```python
from build123d import *
from build123d.topology import SkipClean

# Parameters (mm, degrees)
SKETCH_1_W               = 14
SKETCH_1_H               = 45
EXTRUDE_1_DEPTH          = 3
SKETCH_4_W               = 8
SKETCH_4_H               = 3.5
EXTRUDE_2_DEPTH          = 10
SKETCH_10_W              = 3.5
SKETCH_10_H              = 6
EXTRUDE_3_DEPTH          = 14
CUT_EXTRUDE_1_DEPTH      = 52.078371156
CUT_EXTRUDE_1_DEPTH_BACK = 52.078371156
SKETCH_2_R               = 1.5
SKETCH_3_R               = 3.5
SKETCH_3_R_2             = 1.5
EXTRUDE_1_2_DEPTH        = 5
SKETCH_12_W              = 14
SKETCH_12_H              = 2
EXTRUDE_4_DEPTH          = 5
RIB_9_REACH              = 53.078
SKETCH_13_WALL_W         = 123.475258838
SKETCH_13_WALL_H         = 2.8
RIB_8_REACH              = 53.078
SKETCH_11_WALL_W         = 124.678564032
SKETCH_11_WALL_H         = 3
CHAMFER_3_SIZE           = 0.5
CHAMFER_4_SIZE           = 1
EXTRUDE_5_REACH          = 46.612
EXTRUDE_5_END_RADIUS     = 3.5
SKETCH_15_W              = 5.2
SKETCH_15_H              = 5
CHAMFER_5_SIZE           = 0.606199956
CHAMFER_5_SIZE_2         = 1.3
CUT_EXTRUDE_2_DEPTH      = 4
EXTRUDE_START            = 3
EXTRUDE_6_DEPTH          = 4.393800044
CUT_EXTRUDE_3_DEPTH      = 1
CHAMFER_START            = 2.8
CHAMFER_6_DEPTH          = 2.5
CHAMFER_START_2          = 5.3
CHAMFER_6_2_DEPTH        = 2.7
CHAMFER_START_3          = 3
CHAMFER_6_3_DEPTH        = 3.7
DELETE_START             = 2
DELETE_FACE_1_DEPTH      = 6


with BuildPart() as part:
    # 草图1 → Extrude 1 (new body)
    with BuildSketch(Plane(origin=(0, 0, 0), x_dir=(1, 0, 0), z_dir=(0, 1, 0))):
        with Locations((7, -22.5)):
            Rectangle(SKETCH_1_W, SKETCH_1_H)
    extrude(amount=EXTRUDE_1_DEPTH)

    # 草图4 → 凸台-拉伸2 (add)
    with BuildSketch(Plane.XZ):
        with Locations((18, 1.75)):
            Rectangle(SKETCH_4_W, SKETCH_4_H)
    extrude_2 = extrude(amount=-EXTRUDE_2_DEPTH)

    # 草图9 → 打孔尺寸(%根据)内六角花形半沉头螺钉的类型1 (revolve, cut)
    with BuildSketch(Plane(origin=(18, 5, 3.5), x_dir=(0, -1, 0), z_dir=(1, 0, 0))):
        Polygon((0, 0), (0, 5.96137699), (1.6, 5), (1.6, 1.6), (3.2, 0), align=None)
    hole_wizard_1 = revolve(axis=Axis((18, 5, 9.85), (0, 0, -1)), mode=Mode.SUBTRACT)

    # 镜向1: 凸台-拉伸2, 打孔尺寸(%根据)内六角花形半沉头螺钉的类型1 across plane
    add(extrude_2.mirror(Plane(origin=(7, 0, 0), x_dir=(0, 0, 1), z_dir=(1, 0, 0))))
    add(hole_wizard_1.mirror(Plane(origin=(7, 0, 0), x_dir=(0, 0, 1), z_dir=(1, 0, 0))), mode=Mode.SUBTRACT)

    # 草图10 → 凸台-拉伸3 (add)
    with BuildSketch(Plane.ZY.offset(-14)):
        with Locations((1.75, 6)):
            Rectangle(SKETCH_10_W, SKETCH_10_H)
    extrude(amount=EXTRUDE_3_DEPTH)

    # 草图2 → 切除-拉伸1 (cut, two sides: drawn at the far end of the back side and taken through both)
    with BuildSketch(Plane.XZ.offset(-CUT_EXTRUDE_1_DEPTH_BACK)):
        with Locations(Location((4.5, 41, 0), (0, 0, 270))):
            Circle(SKETCH_2_R)
        with Locations(Location((4.5, 4, 0), (0, 0, 270))):
            Circle(SKETCH_2_R)
    extrude(amount=CUT_EXTRUDE_1_DEPTH + CUT_EXTRUDE_1_DEPTH_BACK, mode=Mode.SUBTRACT)

    # 草图3 → Extrude 1 2 (add)
    # profile 1 of 2: a face of its own
    with SkipClean():  # the faces are left unmerged after this step: merging them gives an invalid solid
        with BuildSketch(Plane(origin=(0, 3, 0), x_dir=(1, 0, 0), z_dir=(0, 1, 0))):
            with Locations((4.5, -41)):
                Circle(SKETCH_3_R)
            with Locations((4.5, -41)):
                Circle(SKETCH_3_R_2, mode=Mode.SUBTRACT)
        # profile 2 of 2: a face of its own
        with BuildSketch(Plane(origin=(0, 3, 0), x_dir=(1, 0, 0), z_dir=(0, 1, 0))):
            with Locations((4.5, -4)):
                Circle(SKETCH_3_R)
            with Locations((4.5, -4)):
                Circle(SKETCH_3_R_2, mode=Mode.SUBTRACT)
        extrude(amount=EXTRUDE_1_2_DEPTH)

    # 草图12 → 凸台-拉伸4 (add)
    with SkipClean():  # the faces are left unmerged after this step: merging them gives an invalid solid
        with BuildSketch(Plane(origin=(0, 3, 0), x_dir=(1, 0, 0), z_dir=(0, 1, 0))):
            with Locations((7, -44)):
                Rectangle(SKETCH_12_W, SKETCH_12_H)
        extrude(amount=EXTRUDE_4_DEPTH)

    # 草图13 wall → 筋9 (add, up to next)
    with BuildSketch(Plane(origin=(14, 5.5, 33.669872981), x_dir=(0, -0.258819045101, -0.96592582629), z_dir=(0, 0.96592582629, -0.258819045101)), mode=Mode.PRIVATE) as rib_9_sk1:
        with Locations((0, 1.4)):
            Rectangle(SKETCH_13_WALL_W, SKETCH_13_WALL_H)
    rib_9_tool1 = extrude(rib_9_sk1.sketch, amount=-RIB_9_REACH, mode=Mode.PRIVATE) - part.part
    rib_9 = rib_9_tool1.solids().sort_by_distance((14, 5.5, 33.669872981))[0]
    add(rib_9)

    # 草图11 wall → 筋8 (add, up to next)
    with BuildSketch(Plane(origin=(14, 6, 13.312557855), x_dir=(0, -0.292371704721, 0.956304755963), z_dir=(0, -0.956304755963, -0.292371704721)), mode=Mode.PRIVATE) as rib_8_sk1:
        with Locations((0, 1.5)):
            Rectangle(SKETCH_11_WALL_W, SKETCH_11_WALL_H)
    rib_8_tool1 = extrude(rib_8_sk1.sketch, amount=RIB_8_REACH, mode=Mode.PRIVATE) - part.part
    rib_8 = rib_8_tool1.solids().sort_by_distance((14, 6, 13.312557855))[0]
    add(rib_8)

    # 镜向2: 筋9, 筋8 across plane
    with SkipClean():  # the faces are left unmerged after this step: merging them gives an invalid solid
        add(rib_9.mirror(Plane(origin=(7, 0, 0), x_dir=(0, 0, 1), z_dir=(1, 0, 0))))
        add(rib_8.mirror(Plane(origin=(7, 0, 0), x_dir=(0, 0, 1), z_dir=(1, 0, 0))))

    # 倒角3
    # the kernel refuses this chamfer: 0.5 mm, written as the material it adds along each edge
    with BuildSketch(Plane(origin=(14, 3, 3.5), x_dir=(1, 0, 0), z_dir=(0, 1, 0))) as chamfer_3_piece_1_section:
        Polygon((CHAMFER_3_SIZE, 0), (0, -CHAMFER_3_SIZE), (0, 0), align=None)
    chamfer_3_piece_1 = extrude(amount=7.285841494, mode=Mode.PRIVATE)
    chamfer_3_piece_1 = split(chamfer_3_piece_1, bisect_by=Plane(origin=(14, 8.487112718, 5.17757871), z_dir=(0, -0.956304755963518, -0.29237170472115837)), keep=Keep.TOP, mode=Mode.PRIVATE)
    add(chamfer_3_piece_1)
    with BuildSketch(Plane(origin=(11, 10.285841494, 3.5), x_dir=(-1, 0, 0), z_dir=(0, -1, 0))) as chamfer_3_piece_2_section:
        Polygon((CHAMFER_3_SIZE, 0), (0, -CHAMFER_3_SIZE), (0, 0), align=None)
    chamfer_3_piece_2 = extrude(amount=8.571682988, mode=Mode.PRIVATE)
    chamfer_3_piece_2 = split(chamfer_3_piece_2, bisect_by=Plane(origin=(11, 9.109915291, 3.140483281), z_dir=(0, -0.956304755963518, -0.29237170472115837)), keep=Keep.TOP, mode=Mode.PRIVATE)
    add(chamfer_3_piece_2)
    with BuildSketch(Plane(origin=(0, 3, 3.5), x_dir=(0, 0, 1), z_dir=(0, 1, 0))) as chamfer_3_piece_3_section:
        Polygon((CHAMFER_3_SIZE, 0), (0, -CHAMFER_3_SIZE), (0, 0), align=None)
    chamfer_3_piece_3 = extrude(amount=7.285841494, mode=Mode.PRIVATE)
    chamfer_3_piece_3 = split(chamfer_3_piece_3, bisect_by=Plane(origin=(0, 8.487112718, 5.17757871), z_dir=(0, -0.956304755963518, -0.29237170472115837)), keep=Keep.TOP, mode=Mode.PRIVATE)
    add(chamfer_3_piece_3)
    with BuildSketch(Plane(origin=(0, 0, 3.5), x_dir=(0, 0, 1), z_dir=(0, 1, 0))) as chamfer_3_piece_4:
        Polygon((CHAMFER_3_SIZE, 0), (0, -CHAMFER_3_SIZE), (0, 0), align=None)
    extrude(amount=3)
    with BuildSketch(Plane(origin=(14, 0, 3.5), x_dir=(0, 0, 1), z_dir=(0, 1, 0))) as chamfer_3_piece_5:
        Polygon((CHAMFER_3_SIZE, 0), (0, CHAMFER_3_SIZE), (0, 0), align=None)
    extrude(amount=3)

    # 倒角4
    chamfer_4_edges = [part.edges().sort_by_distance(p)[0] for p in [
        (-8, 10, 1.75),
        (0, 10, 1.75),
        (14, 10, 1.75),
        (22, 10, 1.75),
    ]]
    chamfer(chamfer_4_edges, length=CHAMFER_4_SIZE - 0.0001)  # a hair under: the kernel refuses the full size

    # 凸台-拉伸5: up to this cylinder (the profile starts outside it)
    extrude_5_end = Plane(origin=(4.5, 5.5, 41), z_dir=(0, -1, 0)) * Cylinder(EXTRUDE_5_END_RADIUS, 101.224, mode=Mode.PRIVATE)
    # 草图15 → 凸台-拉伸5 (add, up to the surface)
    with BuildSketch(Plane(origin=(0, 0, 37.5), x_dir=(-1, 0, 0), z_dir=(0, 0, -1)), mode=Mode.PRIVATE) as extrude_5_sk1:
        with Locations((-5.4, 5.5)):
            Rectangle(SKETCH_15_W, SKETCH_15_H)
    extrude_5_tool1 = extrude(extrude_5_sk1.sketch, amount=-EXTRUDE_5_REACH, mode=Mode.PRIVATE) - extrude_5_end
    add(extrude_5_tool1.solids().sort_by_distance((5.4, 5.5, 37.5))[0])
    add(extrude_5_tool1.solids().sort_by_distance((5.4, 5.5, 37.5))[1])

    # 倒角5
    # the kernel refuses this chamfer: 1.3, 0.606199956 mm, written as the material it takes off along each edge
    with BuildSketch(Plane(origin=(4.5, 8, 37.5), x_dir=(0, -1, 0), z_dir=(1, 0, 0))) as chamfer_5_piece_1:
        Polygon((CHAMFER_5_SIZE, 0), (0, -CHAMFER_5_SIZE_2), (0, 0), align=None)
    extrude(amount=6.868268113, mode=Mode.SUBTRACT)
    with BuildSketch(Plane(origin=(-0.568268113, 8, 37.5), x_dir=(0, -1, 0), z_dir=(1, 0, 0))) as chamfer_5_piece_2:
        Polygon((CHAMFER_5_SIZE, 0), (0, -CHAMFER_5_SIZE_2), (0, 0), align=None)
    extrude(amount=5.068268113, mode=Mode.SUBTRACT)

    # 草图14 → 切除-拉伸2 (cut)
    with BuildSketch(Plane.XZ):
        with BuildLine():
            Line((8.7, 34.5), (8.7, 27.5))
            ThreePointArc((8.7, 27.5), (7, 25.8), (5.3, 27.5))
            Line((5.3, 27.5), (5.3, 34.5))
            ThreePointArc((5.3, 34.5), (7, 36.2), (8.7, 34.5))
        make_face()
        with BuildLine():
            Line((8.7, 10.5), (8.7, 17.5))
            ThreePointArc((8.7, 17.5), (7, 19.2), (5.3, 17.5))
            Line((5.3, 17.5), (5.3, 10.5))
            ThreePointArc((5.3, 10.5), (7, 8.8), (8.7, 10.5))
        make_face()
    extrude(amount=-CUT_EXTRUDE_2_DEPTH, mode=Mode.SUBTRACT)

    # 凸台-拉伸6: read off the stored shape, not the designer's step
    # 凸台-拉伸6 outline → 凸台-拉伸6 (add)
    with BuildSketch(Plane(origin=(0, 0, 0), x_dir=(1, 0, 0), z_dir=(0, 1, 0)).offset(EXTRUDE_START)):
        with BuildLine():
            Line((4.5, -7.5), (8, -7.5))
            Line((8, -7.5), (8, -4))
            ThreePointArc((8, -4), (6.974873734, -6.474873734), (4.5, -7.5))
        make_face()
        with BuildLine():
            Line((3, -7.5), (4.5, -7.5))
            ThreePointArc((4.5, -7.5), (3.731225589, -7.414525722), (3, -7.16227766))
            Line((3, -7.16227766), (3, -7.5))
        make_face()
    extrude(amount=EXTRUDE_6_DEPTH)

    # 草图21 → 切除-拉伸3 (cut)
    with BuildSketch(Plane.XY.offset(7.5)):
        Polygon((3, 7.393800044), (3, 3), (8, 3), (8, 7.393800044), (4.5, 7.393800044), align=None)
    extrude(amount=-CUT_EXTRUDE_3_DEPTH, mode=Mode.SUBTRACT)

    # 倒角6: read off the stored shape, not the designer's step
    # 倒角6 outline → 倒角6 (add)
    with BuildSketch(Plane.YZ.offset(CHAMFER_START)):
        Polygon((3, 6.5), (7.393800044, 6.5), (7.393800044, 7.106199956), (3, 11.5), align=None)
        Polygon((3, 37.5), (3, 32.5), (6.864139677, 36.364139677), (7.393800044, 37.5), align=None)
    extrude(amount=CHAMFER_6_DEPTH)

    # Chamfer 6 2 outline → Chamfer 6 2 (add)
    with BuildSketch(Plane.YZ.offset(CHAMFER_START_2)):
        Polygon((3, 6.5), (7.393800044, 6.5), (7.393800044, 7.106199956), (3, 11.5), align=None)
        Polygon((3, 37.5), (3, 32.5), (6.864139677, 36.364139677), (7.393800044, 37.5), align=None)
    extrude(amount=CHAMFER_6_2_DEPTH)

    # Chamfer 6 3 outline → Chamfer 6 3 (cut)
    with BuildSketch(Plane(origin=(0, 0, 0), x_dir=(1, 0, 0), z_dir=(0, 1, 0)).offset(CHAMFER_START_3)):
        with BuildLine():
            ThreePointArc((8, -9.125227292), (6.228637569, -8.985074259), (5.3, -10.5))
            Line((5.3, -10.5), (5.3, -34.5))
            ThreePointArc((5.3, -34.5), (6.228637569, -36.014925741), (8, -35.874772708))
            Line((8, -35.874772708), (8, -9.125227292))
        make_face()
    extrude(amount=CHAMFER_6_3_DEPTH, mode=Mode.SUBTRACT)

    # Delete Face 1: read off the stored shape, not the designer's step
    # Delete Face 1 outline → Delete Face 1 (add)
    with BuildSketch(Plane(origin=(0, 0, 0), x_dir=(1, 0, 0), z_dir=(0, 1, 0)).offset(DELETE_START)):
        with BuildLine():
            Line((7.372281323, -43), (8, -43))
            Line((8, -43), (8, -41))
            ThreePointArc((8, -41), (7.839385021, -42.048097173), (7.372281323, -43))
        make_face()
    extrude(amount=DELETE_FACE_1_DEPTH)


solid = part.part
```
Geometry check sheet. Reference: the model listing, model coordinates, mm. A direction names the side the tool comes from. Coordinates: 2 decimals unless noted, no trailing zeros. Order: outer loops, then holes, each group sorted by start corner. A loop starts at its lowest first (then second) coordinate and runs counter-clockwise, first axis right, second up. Notation, with made-up numbers: (-5, -32.75) - (35, -32.75) arc R24 cw to (35, 5.25) - close; hole circle Ø7 at (-37.75, -4). An arc over 180 degrees is marked (long way). Answer as a JSON object with one key per item and string values. Group by question number.
Item 1: Tool access check on faces 1 (the face through (2.8, 4, 30)), 2 (the face through (-0.5, 9.5, 1.7)), 3 (the face through (2.8, 6.8, 37)), 4 (the face through (14, 2.7, 23.9)). Record the directions out of +Z, -Z, +X, -X, +Y, -Y that give a thin tool (end or side, any length) a straight path to the whole face; none if there is none.
Item 2: Sectioned sample at A-A, the plane x = -4. Record the cut outline in (y, z).
Item 3: Depth check by flat-ended pin: pin 1 Ø5 at (x, z) = (13, 7) entering from +Y; pin 2 Ø6 at (x, z) = (15, 15) entering from +Y; pin 3 Ø4 at (x, z) = (4.5, 41) entering from +Y. Enter the tip coordinate at first touch or a pass-through.
Item 4: Sectioned sample at C-C, the plane z = 41. Record the cut outline in (x, y), and give its area (3 significant figures).
Item 5: Sectioned sample at B-B, the plane z = 16.5. Record the cut outline in (x, y), and give its area (3 significant figures).
Item 6: Scan lines: probe 1 along X at (y, z) = (3.5, 41); probe 2 along X at (y, z) = (5, 0.7); probe 3 along Z at (x, y) = (4.5, 2). Record each from-to range of solid material in increasing order.
Resolved:
{
 "1": {"face 1": "+Y", "face 2": "+Z, -Z, +Y", "face 3": "-X, +Y", "face 4": "+Z, +X, +Y, -Y"},
 "2": {"outline": "(0, 0) - (3.4, 0) - (3.4, 1.9) - (1.8, 3.5) - (0, 3.5) - close; (6.6, 0) - (10, 0) - (10, 3.5) - (8.2, 3.5) - (6.6, 1.9) - close"},
 "3": {"pin 1": "y = 8.69", "pin 2": "y = 6.35", "pin 3": "y = 8"},
 "4": {"outline": "(0, 0) - (3, 0) - (3, 8) - (1, 8) - (1, 7.46) - (0, 7.46) - close; (6, 0) - (14, 0) - (14, 7.46) - (11.2, 7.46) - (11.2, 3) - (8, 3) - (8, 8) - (6, 8) - close", "area": "70.0 mm^2"},
 "5": {"outline": "(0, 0) - (5.3, 0) - (5.3, 3) - (3, 3) - (3, 5.03) - (0, 5.03) - close; (8.7, 0) - (14, 0) - (14, 5.03) - (11, 5.03) - (11, 3) - (8.7, 3) - close", "area": "44.0 mm^2"},
 "6": {"probe 1": "0 to 3, 6 to 8, 11.2 to 14", "probe 2": "-8 to -5.6, -2.4 to 16.4, 19.6 to 22", "probe 3": "0 to 2.5, 5.5 to 39.5, 42.5 to 45"}
}
